Study the drawing (mm; zero at the part's minimum x, y, z) and answer. Coordinates: 2 decimals unless noted, no trailing zeros. Write each loop counter-clockwise with the first axis right and the second up, starting at its lowest first coordinate (ties: lowest second). Pieces come first, ordered by that corner, then holes. Notation, with made-up numbers: (-9, -27) -> (28, -27) arc R15 ccw to (28, 2) -> close; hole circle Ø4 at (9, 15). An arc over 180 degrees is marked (long way). Answer in a Markdown table with one row per item. Add a question column.
Item 1: Section C-C on z = 1.35 is taken. Write down the section's boundary in (x, y), then the cut area to 3 significant figures.
Item 2: Section D-D on x = 151.5 is taken. Write down the section's boundary in (y, z) (3 decimals), then the cut area to 3 significant figures.
Item 3: Straight lines are drawn through the part: line 1 (Y direction, x = 127, z = 2); line 2 (Y direction, x = 63.5, z = 1.8); line 3 (X direction, y = 26.5, z = 0.2). For each, find the intervals that lie inside material, in ascending order. Write a range as from..to.
Item 4: Section B-B on x = 63.5 is taken. Write down the section's boundary in (y, z) (3 decimals).
Item 5: Section A-A on y = 76.2 is taken. Write down the section's boundary in (x, z) (3 decimals).
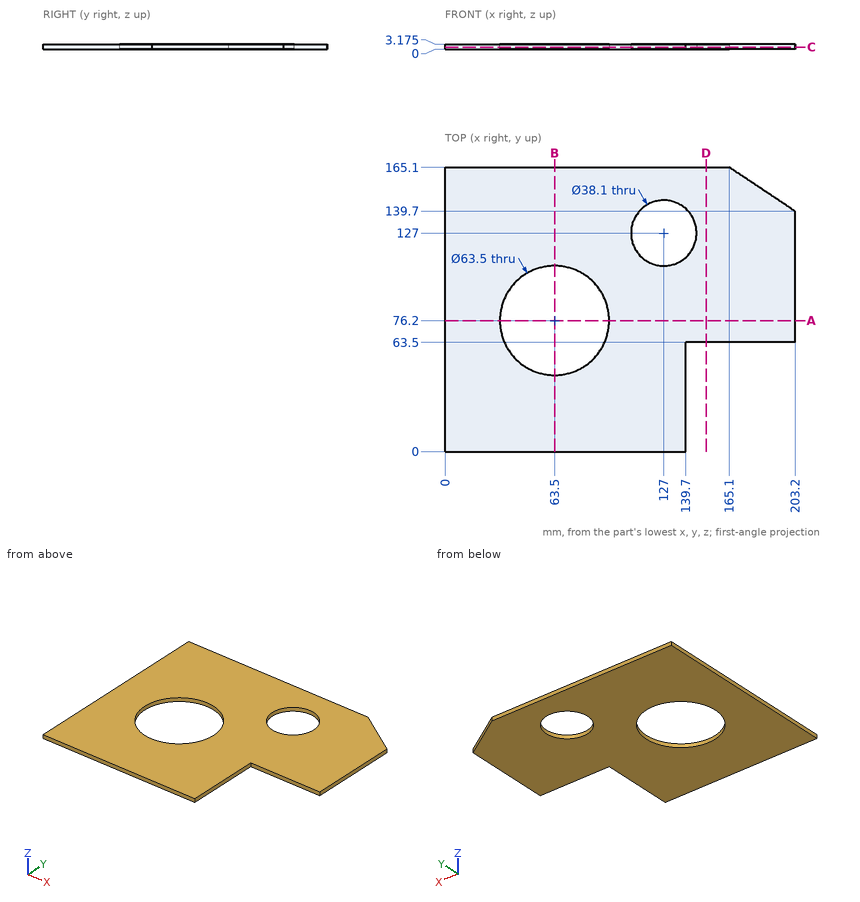
Results below:
| question | item | result |
|---|---|---|
| 1 | outline | (0, 0) -> (139.7, 0) -> (139.7, 63.5) -> (203.2, 63.5) -> (203.2, 139.7) -> (165.1, 165.1) -> (0, 165.1) -> close; hole circle Ø63.5 at (63.5, 76.2); hole circle Ø38.1 at (127, 127) |
| 1 | area | 24,700 mm2 |
| 2 | outline | (63.5, 0) -> (165.1, 0) -> (165.1, 3.175) -> (63.5, 3.175) -> close |
| 2 | area | 323 mm2 |
| 3 | line 1 | y = 0..107.95, 146.05..165.1 |
| 3 | line 2 | y = 0..44.45, 107.95..165.1 |
| 3 | line 3 | x = 0..139.7 |
| 4 | outline | (0, 0) -> (44.45, 0) -> (44.45, 3.175) -> (0, 3.175) -> close; (107.95, 0) -> (165.1, 0) -> (165.1, 3.175) -> (107.95, 3.175) -> close |
| 5 | outline | (0, 0) -> (31.75, 0) -> (31.75, 3.175) -> (0, 3.175) -> close; (95.25, 0) -> (203.2, 0) -> (203.2, 3.175) -> (95.25, 3.175) -> close |
